```python
from build123d import *

# Parameters (mm, degrees)
F0_R     = 125
F2_DEPTH = 10
F1_R     = 15
F3_DEPTH = 39
F4_DEPTH = 107
F5_R     = 8
F7_R     = 18.065377162
F8_DEPTH = 300


# Not quite as in the source:
# - a fillet or chamfer that OpenCascade refuses, or shapes differently, is made with other operations: its cross-section is extruded or revolved along the edge and cut away or added


with BuildPart() as f2:
    # F0 (on Top) → F2 (new body)
    with BuildSketch(Plane.XY):
        Circle(F0_R)
    extrude(amount=F2_DEPTH)

    # F1 (on face) → F3 (join)
    with BuildSketch(Plane.XY):
        with Locations((-45.9619407771, -45.9619407771)):
            Circle(F1_R)
        with Locations((-65, 0)):
            Circle(F1_R)
        with Locations((0, 65)):
            Circle(F1_R)
        with Locations((0, -65)):
            Circle(F1_R)
        with Locations((45.9619407771, -45.9619407771)):
            Circle(F1_R)
        with Locations((65, 0)):
            Circle(F1_R)
        with Locations((45.9619407771, 45.9619407771)):
            Circle(F1_R)
        with Locations((-45.9619407771, 45.9619407771)):
            Circle(F1_R)
    extrude(amount=F3_DEPTH)

    # F4 (cut): faces of the model
    f4_faces = [f2.faces().sort_by_distance(p)[0] for p in [
        (-45.9619407771, -45.9619407771, 39),
        (0, -65, 39),
        (45.9619407771, -45.9619407771, 39),
        (65, 0, 39),
        (45.9619407771, 45.9619407771, 39),
        (0, 65, 39),
        (-45.9619407771, 45.9619407771, 39),
        (-65, 0, 39),
    ]]
    extrude(f4_faces, amount=-F4_DEPTH, mode=Mode.SUBTRACT)

    # F5
    f5_edges = [f2.edges().sort_by_distance(p)[0] for p in [
        (-125, 0, 10),
    ]]
    fillet(f5_edges, radius=F5_R)

    # F6: fillet of radius 8 on 1 edges, made by hand

    # F6_s1 → F6_t2 (revolve, cut)
    with BuildSketch(Plane.XZ):
        with BuildLine():
            ThreePointArc((125, 2), (122.5369245026, 0.5166852265), (119.7084973779, 0))
            Line((119.7084973779, 0), (125, 0))
            Line((125, 0), (125, 2))
        make_face()
    revolve(axis=Axis((0, 0, 0), (0, 0, 1)), mode=Mode.SUBTRACT)

    # F7 (on face) → F8 (join)
    with BuildSketch(Plane(origin=(0, 0, 0), x_dir=(1, 0, 0), z_dir=(0, 0, -1))):
        with Locations((39.3640957773, -86.4013507962)):
            Circle(F7_R)
        with Locations((-86.4013507962, -39.3640957773)):
            Circle(F7_R)
        with Locations((-39.3640957773, 86.4013507962)):
            Circle(F7_R)
        with Locations((86.4013507962, 39.3640957773)):
            Circle(F7_R)
    extrude(amount=F8_DEPTH)


solid = f2.part
```
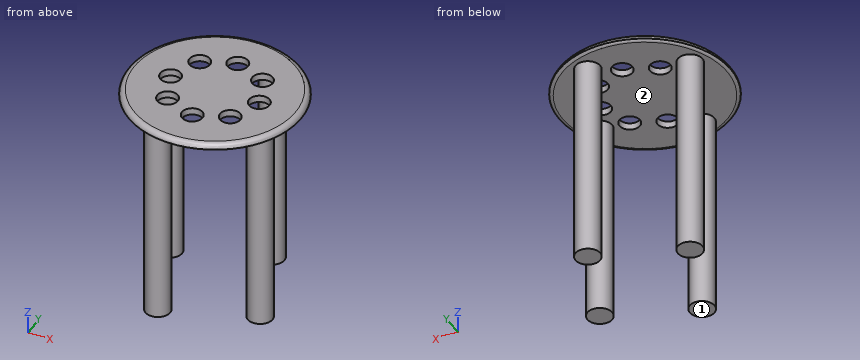
Work out the finished part from the listing and answer in its coordinate system (mm). Face numbers are marked on the shaded views. A direction names the side the tool comes from. Coordinates: 2 decimals unless noted, no trailing zeros. Order: outer loops, then holes, each group sorted by start corner. A loop starts at its lowest first (then second) coordinate and runs counter-clockwise, first axis right, second up. Notation, with made-up numbers: M 62,89 L 106,89 A16 cw 106,110 Z; hole C -10.5,-37 d9. An arc over 180 degrees is marked long. Use CSV: the item, a comma, the result in double quotes.
1) Section A-A on x = 0 is taken. Write down the section's boundary in (y, z), plus the area to 3 significant figures.
Worked out:
outline,"M -125,2 A8 ccw -119.71,0 L -80,0 L -80,10 L -117,10 A8 ccw Z; M -50,0 L 50,0 L 50,10 L -50,10 Z; M 80,0 L 119.71,0 A8 ccw 125,2 A8 ccw 117,10 L 80,10 Z"
area,"1,870 mm^2"
2) Section C-C on z = -168 is taken. Write down the section's boundary in (x, y), plus the area to 3 significant figures.
Worked out:
outline,"C -86.4,39.36 d36.13; C -39.36,-86.4 d36.13; C 39.36,86.4 d36.13; C 86.4,-39.36 d36.13"
area,"4,100 mm^2"
3) For the marked faces 1 and 2, determine the directions among +Z, -Z, +X, -X, +Y, -Y from which every point of the face is accessible in a straight line to the end or side of a thin tool.
Worked out:
face 1,"-Z, +X, -X, +Y, -Y"
face 2,"-Z"
4) Consider line 1 (Y direction, x = 0, z = 2); line 2 (Z direction, x = -62, y = -64); line 3 (X direction, y = 39, z = -199.5). Determine where each line is inside the solid, lowest interval first. Write a range as [from, to].
Worked out:
line 1,"y = [-125, -80], [-50, 50], [80, 125]"
line 2,"z = [0, 10]"
line 3,"x = [-104.46, -68.34]"
5) Flat-ended cylindrical pins translate along their axes: pin 1 Ø5 at (x, z) = (-88, -29) entering from -Y; pin 2 Ø3 at (x, z) = (98, -182.5) entering from -Y; pin 3 Ø8 at (x, z) = (-30.5, -94) entering from -Y; pin 4 Ø24 at (x, y) = (-45.96, 45.96) entering from +Z. Find the tip coordinate at first contact, or state that the pin passes through.
Worked out:
pin 1,"stops at y = 21.3"
pin 2,"stops at y = -54.34"
pin 3,"stops at y = -103.8"
pin 4,"passes through"
6) Section D-D on x = 41.5 is taken. Count the separate pieces of the cut face and the enclosed holes in it, plus the area to 3 significant figures.
Worked out:
separate pieces,"3"
enclosed holes,"0"
area,"12,500 mm^2"
